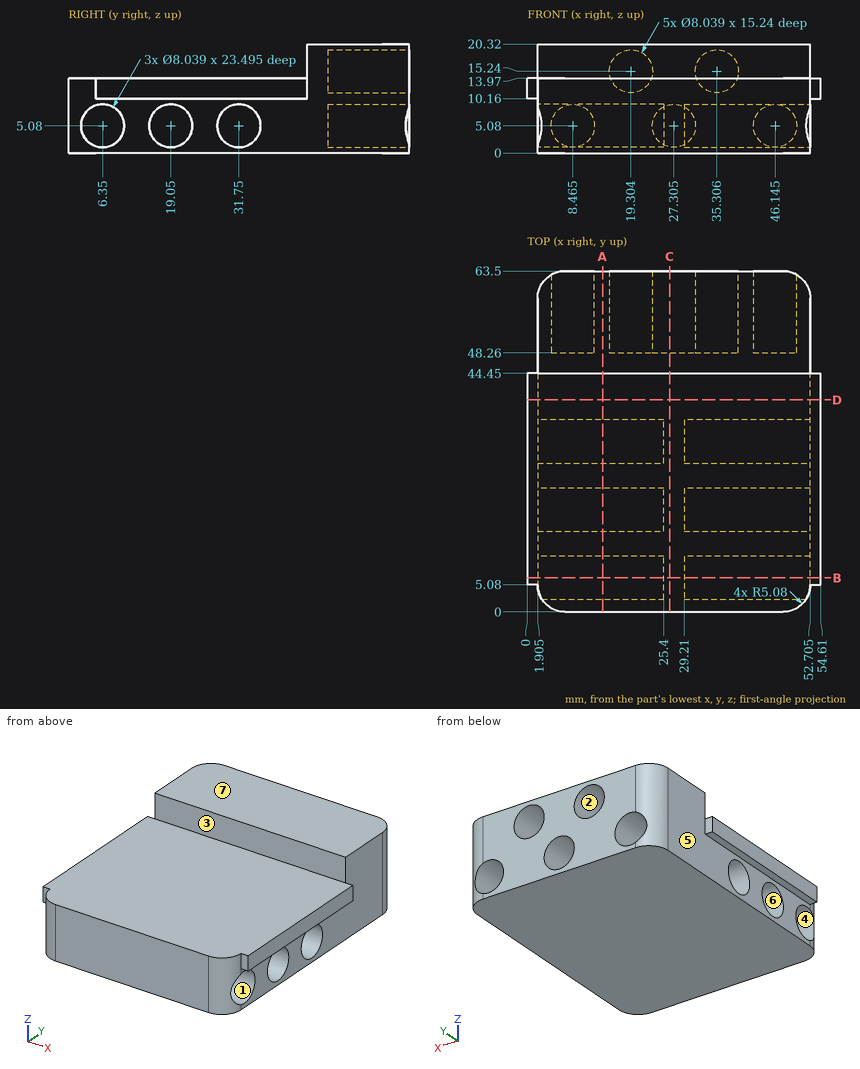
Study the drawing (mm; zero at the part's minimum x, y, z) and answer. A direction names the side the tool comes from. Round coordinates to 2 decimals unless told otherwise and drop trailing zeros. Write each loop counter-clockwise with the first axis right and the second up, starting at its lowest first coordinate (ties: lowest second). Pieces come first, ordered by that corner, then holes.
1) A cutting plane is placed at A-A on x = 14. Determine the outline of the cut face in (y, z), and give its area (3 significant figures).
2) A cutting plane is placed at C-C on x = 26.5. Determine the outline of the cut face in (y, z).
3) Consider probe 1 along Y at (x, z) = (43, 4.75) (1 decimal); probe 2 along Y at (x, z) = (49, 7.25) (1 decimal); probe 3 along X at (y, z) = (60.5, 4.25). Determine where each line is inside the solid, lowest interval first.
4) Determine the mould class of the marked faces 5, 6 and 7 for opening direction Z: pulls with the +Z half, pulls with the -Z half, needs draft (parallel to the pull), parting line crosses it, or undercut.
5) A cutting plane is placed at B-B on y = 6.35. Determine the outline of the cut face in (x, z) (1 decimal).
6) Flat-ended cylindrical pins translate along their axes: P1, Ø0.6, axis at x = 1.5, y = 20.5, coming from the -Z side; P2, Ø2, axis at y = 46.5, z = 13.5, coming from the +X side (3 decimals); P3, Ø6.5, axis at y = 6.35, z = 5.08, coming from the -X side. Find the tip coordinate at first contact, or state that the pin passes through.
7) A cutting plane is placed at D-D on y = 39.5. Determine the outline of the cut face in (x, z) (1 decimal), and give its area (3 significant figures).
8) Which of the six approach directions +Z, -Z, +X, -X, +Y, -Y give full straight-line access (tool end or side, diameter ignored) to the marked faces 1, 2, 3 and 4?
Entries:
1. outline: (0, 0) - (63.5, 0) - (63.5, 20.32) - (44.45, 20.32) - (44.45, 13.97) - (0, 13.97) - close; hole circle Ø8.04 at (6.35, 5.08); hole circle Ø8.04 at (19.05, 5.08); hole circle Ø8.04 at (31.75, 5.08)
1. area: 856 mm2
2. outline: (0, 0) - (63.5, 0) - (63.5, 1.14) - (48.26, 1.14) - (48.26, 9.02) - (63.5, 9.02) - (63.5, 20.32) - (44.45, 20.32) - (44.45, 13.97) - (0, 13.97) - close
3. probe 1: y = 0 to 2.3, 10.4 to 15, 23.1 to 27.7, 35.8 to 48.3
3. probe 2: y = 0.2 to 3, 9.7 to 15.7, 22.4 to 28.4, 35.1 to 48.3
3. probe 3: x = 2.35 to 4.53, 12.4 to 23.37, 31.24 to 42.21, 50.08 to 52.26
4. face 5: needs draft
4. face 6: undercut
4. face 7: pulls with the +Z half
5. outline: (0, 10.2) - (1.9, 10.2) - (1.9, 9.1) - (25.4, 9.1) - (25.4, 1.1) - (1.9, 1.1) - (1.9, 0) - (52.7, 0) - (52.7, 1.1) - (29.2, 1.1) - (29.2, 9.1) - (52.7, 9.1) - (52.7, 10.2) - (54.6, 10.2) - (54.6, 14) - (0, 14) - close
6. P1: stops at z = 10.16
6. P2: stops at x = 52.705
6. P3: stops at x = 25.4
7. outline: (0, 10.2) - (1.9, 10.2) - (1.9, 0) - (52.7, 0) - (52.7, 10.2) - (54.6, 10.2) - (54.6, 14) - (0, 14) - close
7. area: 724 mm2
8. face 1: +X
8. face 2: +Y
8. face 3: +Z, +X, -X, -Y
8. face 4: -X
